from build123d import *

# Parameters (mm, degrees)
SKETCH2_R           = 2.1
SKETCH2_W           = 72
SKETCH2_H           = 43
BOSS_EXTRUDE1_DEPTH = 10
SKETCH3_W           = 78
SKETCH3_H           = 49
SKETCH3_R           = 2.6
BOSS_EXTRUDE2_DEPTH = 2
SKETCH4_R           = 0.75
CUT_EXTRUDE1_DEPTH  = 10


with BuildPart() as part:
    # Sketch2 → Boss-Extrude1 (new body)
    with BuildSketch(Plane(origin=(0, 0, 0), x_dir=(1, 0, 0), z_dir=(0, 1, 0))):
        with BuildLine():
            Line((-39, 24.5), (-39, 10.89))
            Line((-39, 10.89), (-39, -10.89))
            Line((-39, -10.89), (-39, -24.5))
            Line((-39, -24.5), (-10.89, -24.5))
            ThreePointArc((-10.89, -24.5), (0, -35.39), (10.89, -24.5))
            Line((10.89, -24.5), (39, -24.5))
            Line((39, -24.5), (39, -10.89))
            Line((39, -10.89), (39, 10.89))
            Line((39, 10.89), (39, 24.5))
            Line((39, 24.5), (10.89, 24.5))
            ThreePointArc((10.89, 24.5), (0, 35.39), (-10.89, 24.5))
            Line((-10.89, 24.5), (-39, 24.5))
        make_face()
        with Locations(Location((0, 29.5, 0), (0, 0, 270))):
            Circle(SKETCH2_R, mode=Mode.SUBTRACT)
        with Locations(Location((0, -29.5, 0), (0, 0, 270))):
            Circle(SKETCH2_R, mode=Mode.SUBTRACT)
        Rectangle(SKETCH2_W, SKETCH2_H, mode=Mode.SUBTRACT)
    extrude(amount=BOSS_EXTRUDE1_DEPTH)

    # Sketch3 → Boss-Extrude2 (add)
    with BuildSketch(Plane(origin=(0, 10, 0), x_dir=(1, 0, 0), z_dir=(0, 1, 0))):
        Rectangle(SKETCH3_W, SKETCH3_H)
        with Locations(Location((-24, 18.5, 0), (0, 0, 270))):
            Circle(SKETCH3_R, mode=Mode.SUBTRACT)
        with Locations(Location((-14, 18.5, 0), (0, 0, 270))):
            Circle(SKETCH3_R, mode=Mode.SUBTRACT)
        with Locations(Location((-4, 18.5, 0), (0, 0, 270))):
            Circle(SKETCH3_R, mode=Mode.SUBTRACT)
        with Locations(Location((6, 18.5, 0), (0, 0, 270))):
            Circle(SKETCH3_R, mode=Mode.SUBTRACT)
        with Locations(Location((16, 18.5, 0), (0, 0, 270))):
            Circle(SKETCH3_R, mode=Mode.SUBTRACT)
        with Locations(Location((26, 18.5, 0), (0, 0, 270))):
            Circle(SKETCH3_R, mode=Mode.SUBTRACT)
    extrude(amount=BOSS_EXTRUDE2_DEPTH)

    # Sketch4 → Cut-Extrude1 (cut)
    with BuildSketch(Plane(origin=(0, 12, 0), x_dir=(1, 0, 0), z_dir=(0, 1, 0))):
        with Locations(Location((23, 6.5, 0), (0, 0, 270))):
            Circle(SKETCH4_R)
    extrude(amount=-CUT_EXTRUDE1_DEPTH, mode=Mode.SUBTRACT)


solid = part.part
Source: CAD feature listing. Evaluate the final solid. Frame: model axes, mm. A direction names the side the tool comes from. Give positions to 0.01 mm unless a question says otherwise; leave off trailing zeros. Write each loop counter-clockwise with the first axis right and the second up, starting at its lowest first coordinate (ties: lowest second). Pieces come first, ordered by that corner, then holes. Notation, with made-up numbers: M -19.75,-2 L 29.25,-2 A14 ccw 29.25,15 Z; hole C 61,73 d7. An arc over 180 degrees is marked long. Return JSON: item names as keys, results as strings. Group by question number.
1) Draft query along Z for faces 4 (the face through (-1, 11, -24.5)), 5 (the face through (-36, 5, 0)), 6 (the face through (-1, 12, 0)). Return one class per face: released by +Z, released by -Z, zero draft, split by the parting line, or undercut.
2) Set-up query: faces 1 (the face through (36, 5, 0)), 2 (the face through (-3, 10, -29)), 3 (the face through (28.578, 10.986, -18.838)). Return all of +Z, -Z, +X, -X, +Y, -Y with unobstructed straight access to the full face (end or side cutting, diameter ignored); none if empty.
3) Cut plane D-D, the plane z = 2.5. Output: boundary loops of the cut face in (x, y).
4) Cut plane C-C, the plane x = 16. Output: boundary loops of the cut face in (y, z).
5) First-contact query: pin 1 Ø3.5 at (x, y) = (-18.5, 6.5) entering from +Z; pin 2 Ø13 at (x, z) = (-1, -9) entering from -Y; pin 3 Ø5.5 at (x, z) = (1.5, -31.5) entering from +Y. Flat tips, straight axial feed; report the tip coordinate or a pass-through.
6) Ray query, L1, parallel to Z at x = -18.5, y = 9.25; L2, parallel to X at y = 1.5, z = -5; L3, parallel to X at y = 11.05, z = -6.5. Return the intervals inside material, ascending.
7) Cut plane A-A, the plane x = 0. Output: boundary loops of the cut face in (y, z), then the cut area to 3 significant figures.
8) Cut plane B-B, the plane y = 6. Output: boundary loops of the cut face in (x, z), then the cut area to 3 significant figures.
Data:
{
 "1": {"face 4": "released by -Z", "face 5": "undercut", "face 6": "zero draft"},
 "2": {"face 1": "-Y", "face 2": "-Z, +X, -X, +Y", "face 3": "+Y, -Y"},
 "3": {"outline": "M -39,0 L -36,0 L -36,10 L 36,10 L 36,0 L 39,0 L 39,12 L -39,12 Z"},
 "4": {"outline": "M 0,-24.5 L 12,-24.5 L 12,-21.1 L 10,-21.1 L 10,-21.5 L 0,-21.5 Z; M 0,21.5 L 10,21.5 L 10,-15.9 L 12,-15.9 L 12,24.5 L 0,24.5 Z"},
 "5": {"pin 1": "stops at z = 24.5", "pin 2": "stops at y = 10", "pin 3": "stops at y = 10"},
 "6": {"L1": "z = -24.5 to -21.5, 21.5 to 24.5", "L2": "x = -39 to -36, 36 to 39", "L3": "x = -39 to 22.25, 23.75 to 39"},
 "7": {"outline": "M 0,-35.39 L 10,-35.39 L 10,-31.6 L 0,-31.6 Z; M 0,-27.4 L 10,-27.4 L 10,-24.5 L 12,-24.5 L 12,24.5 L 10,24.5 L 10,27.4 L 0,27.4 L 0,21.5 L 10,21.5 L 10,-21.5 L 0,-21.5 Z; M 0,31.6 L 10,31.6 L 10,35.39 L 0,35.39 Z", "area": "292 mm²"},
 "8": {"outline": "M -39,-24.5 L -10.89,-24.5 A10.89 ccw 10.89,-24.5 L 39,-24.5 L 39,24.5 L 10.89,24.5 A10.89 ccw -10.89,24.5 L -39,24.5 Z; hole M -36,-21.5 L 36,-21.5 L 36,21.5 L -36,21.5 Z; hole C 0,-29.5 d4.2; hole C 0,29.5 d4.2", "area": "1,070 mm²"}
}
